from build123d import *

# Parameters (mm, degrees)
SKETCH1_W                      = 30
SKETCH1_H                      = 40
BASE_FLANGE1_DEPTH             = 0.7366
EDGE_FLANGE1_STRIP_W           = 4.4196
EDGE_FLANGE1_STRIP_H           = 0.7366
EDGE_FLANGE1_STRIP_CUT_DEPTH   = 40
EDGE_FLANGE1_STRIP_2_W         = 4.4196
EDGE_FLANGE1_STRIP_2_H         = 0.7366
EDGE_FLANGE1_STRIP_CUT_2_DEPTH = 40
EDGE_FLANGE1_DEPTH             = 40
EDGE_FLANGE1_BEND_DEPTH        = 40
HEM1_START                     = -20
HEM1_DEPTH                     = 40
HEM1_2_DEPTH                   = 40
F_7_1_7_1_DIAMETER_HOLE1_D     = 7.1


# Read off the part's stored shape, not the designer's step: Hem1
# Sheet-metal steps are written as plain solids
with BuildPart() as part:
    # Sketch1 → Base-Flange1 (new body)
    with BuildSketch(Plane(origin=(0, 0, 0), x_dir=(1, 0, 0), z_dir=(0, 1, 0))):
        Rectangle(SKETCH1_W, SKETCH1_H)
    extrude(amount=-BASE_FLANGE1_DEPTH)

    # Edge-Flange1 strip (across the edge) → Edge-Flange1 strip cut (cut)
    with BuildSketch(Plane(origin=(15, 0, 20), x_dir=(-1, 0, 0), z_dir=(0, 0, -1))):
        with Locations((-1.4732, -0.3683)):
            Rectangle(EDGE_FLANGE1_STRIP_W, EDGE_FLANGE1_STRIP_H)
    extrude(amount=EDGE_FLANGE1_STRIP_CUT_DEPTH, mode=Mode.SUBTRACT)

    # Edge-Flange1 strip 2 (across the edge) → Edge-Flange1 strip cut 2 (cut)
    with BuildSketch(Plane(origin=(-15, 0, -20), x_dir=(1, 0, 0), z_dir=(0, 0, 1))):
        with Locations((-1.4732, -0.3683)):
            Rectangle(EDGE_FLANGE1_STRIP_2_W, EDGE_FLANGE1_STRIP_2_H)
    extrude(amount=EDGE_FLANGE1_STRIP_CUT_2_DEPTH, mode=Mode.SUBTRACT)

    # Edge-Flange1 section (across the edge) → Edge-Flange1 (add)
    with BuildSketch(Plane(origin=(15, 0, 20), x_dir=(-1, 0, 0), z_dir=(0, 0, -1))):
        with BuildLine():
            Line((-0.7366, 0.7366), (-0.7366, 45))
            Line((-0.7366, 45), (0, 45))
            Line((0, 45), (0, 0.7366))
            ThreePointArc((0, 0.7366), (0.215745145, 0.215745145), (0.7366, 0))
            Line((0.7366, 0), (0.7366, -0.7366))
            ThreePointArc((0.7366, -0.7366), (-0.30510971, -0.30510971), (-0.7366, 0.7366))
        make_face()
    extrude(amount=EDGE_FLANGE1_DEPTH)

    # Edge-Flange1 section 2 (across the edge) → Edge-Flange1 bend (add)
    with BuildSketch(Plane(origin=(-15, 0, -20), x_dir=(1, 0, 0), z_dir=(0, 0, 1))):
        with BuildLine():
            Line((-0.7366, 0.7366), (-0.7366, 45))
            Line((-0.7366, 45), (0, 45))
            Line((0, 45), (0, 0.7366))
            ThreePointArc((0, 0.7366), (0.215745145, 0.215745145), (0.7366, 0))
            Line((0.7366, 0), (0.7366, -0.7366))
            ThreePointArc((0.7366, -0.7366), (-0.30510971, -0.30510971), (-0.7366, 0.7366))
        make_face()
    extrude(amount=EDGE_FLANGE1_BEND_DEPTH)

    # Hem1 outline → Hem1 (cut)
    with BuildSketch(Plane.XY.offset(HEM1_START)):
        with BuildLine():
            ThreePointArc((15, 44.2134), (15.212984467, 44.751642306), (15.7366, 44.998409274))
            Line((15.7366, 44.998409274), (15.7366, 45))
            Line((15.7366, 45), (15, 45))
            Line((15, 45), (15, 44.2134))
        make_face()
        with BuildLine():
            Line((-15.7366, 45), (-15.7366, 44.998409274))
            ThreePointArc((-15.7366, 44.998409274), (-15.212984467, 44.751642306), (-15, 44.2134))
            Line((-15, 44.2134), (-15, 45))
            Line((-15, 45), (-15.7366, 45))
        make_face()
    extrude(amount=HEM1_DEPTH, mode=Mode.SUBTRACT)

    # Hem1 2 outline → Hem1 2 (add)
    with BuildSketch(Plane.XY.offset(HEM1_START)):
        with BuildLine():
            Line((15.8366, 0), (16.5732, 0))
            Line((16.5732, 0), (16.5732, 44.2134))
            ThreePointArc((16.5732, 44.2134), (16.324842306, 44.787015533), (15.7366, 44.998409274))
            Line((15.7366, 44.998409274), (15.7366, 44.2134))
            ThreePointArc((15.7366, 44.2134), (15.7866, 44.2634), (15.8366, 44.2134))
            Line((15.8366, 44.2134), (15.8366, 0))
        make_face()
        with BuildLine():
            Line((-16.5732, 0), (-15.8366, 0))
            Line((-15.8366, 0), (-15.8366, 44.2134))
            ThreePointArc((-15.8366, 44.2134), (-15.7866, 44.2634), (-15.7366, 44.2134))
            Line((-15.7366, 44.2134), (-15.7366, 44.998409274))
            ThreePointArc((-15.7366, 44.998409274), (-16.324842306, 44.787015533), (-16.5732, 44.2134))
            Line((-16.5732, 44.2134), (-16.5732, 0))
        make_face()
    extrude(amount=HEM1_2_DEPTH)

    # Ø7.1 (7.1) Diameter Hole1 (through all)
    with Locations(Plane(origin=(16.5732, 0, 0), x_dir=(0, 0, -1), z_dir=(1, 0, 0))):
        with Locations((0, 29.2134)):
            Hole(F_7_1_7_1_DIAMETER_HOLE1_D / 2)


solid = part.part
Design review of the part built by this model. Coordinates are the model's own, in mm. A direction names the side the tool comes from. Coordinates: 2 decimals unless noted, no trailing zeros. Order: outer loops, then holes, each group sorted by start corner. A loop starts at its lowest first (then second) coordinate and runs counter-clockwise, first axis right, second up.
Item 1: For line 1 (Y direction, x = 13, z = 0.5); line 2 (Y direction, x = 16.1, z = 0); line 3 (Y direction, x = -15.15, z = 0), list the stretches that pass through material, from the lowest coordinate up.
Item 2: Take a section at C-C, the plane z = 0. Count the separate pieces of the cut face and the enclosed holes in it, then the cut area to 3 significant figures.
Item 3: For pin 1 Ø5.5 at (y, z) = (29.21, 0) entering from +X; pin 2 Ø3 at (x, z) = (-6, 10.5) entering from +Y; pin 3 Ø0.6 at (x, z) = (16, -5.5) entering from -Y, all flat-tipped, find the tip position at first contact; note any pin that passes through.
Item 4: The part is to be moulded in two halves that separate along Y. For faces 1 (the flat face through (-16.573, 22, 0)), 2 (the cylindrical face through (-15.29, -0.32, -0.28)), 3 (the cylindrical face through (-15.373, 32.733, -0.462)), 4 (the flat face through (0, 0, 0)), say which applies: pulls with the +Y half, pulls with the -Y half, needs draft (parallel to the pull), parting line crosses it, or undercut.
Item 5: For faces 5 (the cylindrical face through (15.363, 32.733, -0.462)), 6 (the flat face through (15, 23, 0)), 7 (the cylindrical face through (15.29, -0.32, 0.28)), list the 3-axis set-ups (+Z, -Z, +X, -X, +Y, -Y) from which the entire face can be reached by the end or side of a thin tool; tool diameter is ignored.
Item 6: Take a section at D-D, the plane x = 0. Write out the cut boundary in (y, z), then the cut area to 3 significant figures.
Item 7: Take a section at B-B, the plane z = 5.5. Write out the cut boundary in (x, y).
Item 8: Take a section at A-A, the plane y = 11. Write out the cut boundary in (x, z).
The answers:
1. line 1: y = -0.74 to 0
1. line 2: y = 0 to 25.66, 32.76 to 44.93
1. line 3: y = -0.44 to 25.66, 32.76 to 44.68
2. separate pieces: 5
2. enclosed holes: 0
2. area: 134 mm2
3. pin 1: passes through
3. pin 2: stops at y = 0
3. pin 3: stops at y = 0
4. face 1: needs draft
4. face 2: pulls with the -Y half
4. face 3: undercut
4. face 4: pulls with the +Y half
5. face 5: +X, -X
5. face 6: +Z, -Z, +Y
5. face 7: +Z, -Z, -Y
6. outline: (-0.74, -20) - (0, -20) - (0, 20) - (-0.74, 20) - close
6. area: 29.5 mm2
7. outline: (-16.57, 0) - (-15.84, 0) - (-15.84, 44.21) arc R0.05 cw to (-15.74, 44.21) - (-15.74, 0.74) arc R1.47 ccw to (-14.26, -0.74) - (14.26, -0.74) arc R1.47 ccw to (15.74, 0.74) - (15.74, 44.21) arc R0.05 cw to (15.84, 44.21) - (15.84, 0) - (16.57, 0) - (16.57, 44.21) arc R0.79 ccw to (15, 44.21) - (15, 0.74) arc R0.74 cw to (14.26, 0) - (-14.26, 0) arc R0.74 cw to (-15, 0.74) - (-15, 44.21) arc R0.79 ccw to (-16.57, 44.21) - close
8. outline: (-16.57, -20) - (-15.84, -20) - (-15.84, 20) - (-16.57, 20) - close; (-15.74, -20) - (-15, -20) - (-15, 20) - (-15.74, 20) - close; (15, -20) - (15.74, -20) - (15.74, 20) - (15, 20) - close; (15.84, -20) - (16.57, -20) - (16.57, 20) - (15.84, 20) - close
